The listing builds one solid part. Answer for the finished solid, in the listing's coordinates (mm). Face numbers are marked on the shaded views. A direction names the side the tool comes from. Give positions to 0.01 mm unless a question says otherwise; leave off trailing zeros. Order: outer loops, then holes, each group sorted by start corner. A loop starts at its lowest first (then second) coordinate and runs counter-clockwise, first axis right, second up. Notation, with made-up numbers: (13, 69.5) - (17, 69.5) arc R16 cw to (17, 90.5) - close; hole circle Ø9 at (-17.5, 47). An arc over 180 degrees is marked (long way). Answer as CSV lines item,"result". Start each with the question number.
1. Section C-C on x = -3.5 is taken. Give the vertices of the cut face in (y, z).
2. Section D-D on z = 18.25 is taken. Give the vertices of the cut face in (x, y).
3. Section B-B on z = 9.5 is taken. Give the vertices of the cut face in (x, y), and give its area (3 significant figures).
4. Flat-ended cylindrical pins translate along their axes: pin 1 (12 mm diameter, centred on x = -16, y = -15, fed in from +Z); pin 2 (2 mm diameter, centred on y = 11.5, z = 19.5, fed in from +X); pin 3 (4 mm diameter, centred on x = 30.5, z = 17, fed in from -Y). Find the tip coordinate at first contact, or state that the pin passes through.
5. Consider line 1 along Z through (x, y) = (1, 6); line 2 along Y through (x, z) = (33, 11); line 3 along X through (y, z) = (-11, 10.75). Determine where each line is inside the solid, lowest interval first. Write a range as [from, to].
6. Which of the six approach directions +Z, -Z, +X, -X, +Y, -Y give full straight-line access (tool end or side, diameter ignored) to the marked faces 1 and 2?
7. Section A-A on y = 9 is taken. Give the vertices of the cut face in (x, z), and give its area (3 significant figures).
8. Determine the mould class of the marked faces 3, 4 and 5 for opening direction X: +X half, -X half, draft (parallel to the pull), parting line (faces both ways), or undercut.
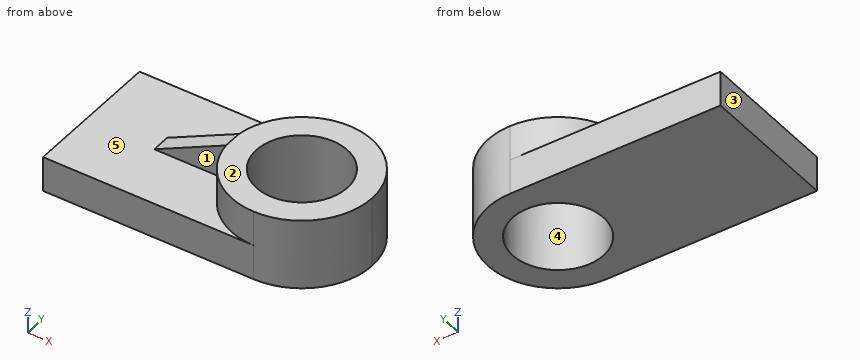
from build123d import *

# Parameters (mm, degrees)
F0_R     = 16.413016
F1_DEPTH = 25.4
F2_DEPTH = 12.7
F4_DEPTH = 12.7
F6_DEPTH = 508


with BuildPart() as f1:
    # F0 (on Top) → F1 (new body)
    with BuildSketch(Plane.XY):
        with BuildLine():
            ThreePointArc((38.069274, 25.34879), (12.720484, 0), (38.069274, -25.34879))
            ThreePointArc((38.069274, -25.34879), (55.993576, -17.924301), (63.418064, 0))
            ThreePointArc((63.418064, 0), (55.993576, 17.924301), (38.069274, 25.34879))
        make_face()
        with Locations((38.069274, 0)):
            Circle(F0_R, mode=Mode.SUBTRACT)
    extrude(amount=F1_DEPTH)

    # F0 (on Top) → F2 (join)
    with BuildSketch(Plane.XY):
        with BuildLine():
            Line((-38.069274, 25.34879), (-38.069274, -25.34879))
            Line((-38.069274, -25.34879), (38.069274, -25.34879))
            ThreePointArc((38.069274, -25.34879), (12.720484, 0), (38.069274, 25.34879))
            Line((38.069274, 25.34879), (-38.069274, 25.34879))
        make_face()
    extrude(amount=F2_DEPTH)

    # F3 (on face) → F4 (join)
    with BuildSketch(Plane.XY.offset(12.7)):
        with BuildLine():
            ThreePointArc((12.950446, -3.406704), (12.720484, 0), (12.950446, 3.406704))
            Line((12.950446, 3.406704), (-12.950446, 3.406704))
            Line((-12.950446, 3.406704), (-12.950446, -3.406704))
            Line((-12.950446, -3.406704), (12.950446, -3.406704))
        make_face()
    extrude(amount=F4_DEPTH)

    # F5 (on face) → F6 (cut)
    with BuildSketch(Plane.XZ.offset(3.406704)):
        Polygon((-12.950446, 25.4), (-12.950446, 12.7), (12.950446, 25.4), align=None)
    extrude(amount=-F6_DEPTH, mode=Mode.SUBTRACT)


solid = f1.part
Checks:
1,outline,"(-25.35, 0) - (25.35, 0) - (25.35, 12.7) - (3.41, 12.7) - (3.41, 17.33) - (-3.41, 17.33) - (-3.41, 12.7) - (-25.35, 12.7) - close"
2,outline,"(-1.63, -3.41) - (12.95, -3.41) arc R25.35 ccw (long way) to (12.95, 3.41) - (-1.63, 3.41) - close; hole circle Ø32.83 at (38.07, 0)"
3,outline,"(-38.07, -25.35) - (38.07, -25.35) arc R25.35 ccw to (63.42, 0) arc R25.35 ccw to (38.07, 25.35) - (-38.07, 25.35) - close; hole circle Ø32.83 at (38.07, 0)"
3,area,"4,020 mm²"
4,pin 1,"stops at z = 12.7"
4,pin 2,"stops at x = 61.14"
4,pin 3,"stops at y = -24.73"
5,line 1,"z = [0, 12.7]"
5,line 2,"y = [-25.35, -15.61], [15.61, 25.35]"
5,line 3,"x = [-38.07, 25.89], [50.25, 60.91]"
6,face 1,"+Z, -X, -Y"
6,face 2,"+Z, +X, -X, +Y, -Y"
7,outline,"(-38.07, 0) - (24.34, 0) - (24.34, 25.4) - (14.37, 25.4) - (14.37, 12.7) - (-38.07, 12.7) - close; (51.79, 0) - (61.77, 0) - (61.77, 25.4) - (51.79, 25.4) - close"
7,area,"1,170 mm²"
8,face 3,"-X half"
8,face 4,"undercut"
8,face 5,"draft"
